For this review, take the finished solid that the model builds, in its own axes (mm). Face numbers are marked on the shaded views. Coordinates: 2 decimals unless noted, no trailing zeros. Loops run counter-clockwise (first coordinate to the right, second up) from the corner with the lowest first, then second, coordinate; pieces in that order, holes last. Notation, with made-up numbers: M 62,40 L 95,40 A33 ccw 95,75 Z; hole C 58,-25 d10. An arc over 180 degrees is marked long. Use one line per item in the form item = value.
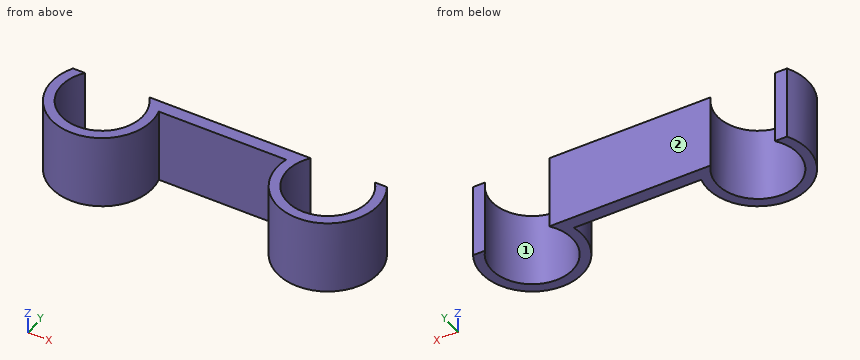
Autodesk Fusion 360 part; units mm, degrees
sketch "スケッチ1" plane through (0, 0, 0) normal (0, 0, 1) x (1, 0, 0)
  arc A0 (-11.5217, 2) -> (-4.0754, 1) centre (-8, 0) ccw
  arc A1 (-10.5617, 2) -> (-5.4383, 2) centre (-8, 0) ccw
  line L0 (-11.5217, 2) -> (-10.5617, 2)
  line L1 (-6, 1) -> (-4.9077, 1)
  line L2 (-4.0754, 1) -> (6.0754, 1)
  arc A2 (6.0754, 1) -> (13.5217, 2) centre (10, 0) ccw
  arc A3 (7.4383, 2) -> (12.5617, 2) centre (10, 0) ccw
  line L3 (-5.4383, 2) -> (7.4383, 2)
  line L4 (12.5617, 2) -> (13.5217, 2)
  dimension "d7" = 6.5
  dimension "d8" = 6.5
extrude "押し出し3" add sketch "スケッチ1" along normal blind 6
extrude "押し出し2" [suppressed]
1. Consider section D-D on x = 10. Write out the cut boundary in (y, z).
Computed values:
outline = M -4.05,0 L -3.25,0 L -3.25,6 L -4.05,6 Z
2. Draft analysis for pull direction X (two halves, no side actions). For the marked faces 1 and 2, state which applies: +X half, -X half, draft (parallel to the pull), parting line (faces both ways), or undercut.
Computed values:
face_1 = undercut
face_2 = draft
3. Consider section C-C on y = 1.5. Write out the cut boundary in (x, z), plus the area to 3 significant figures.
Computed values:
outline = M -11.76,0 L -10.88,0 L -10.88,6 L -11.76,6 Z; M -5.12,0 L 7.12,0 L 7.12,6 L -5.12,6 Z; M 12.88,0 L 13.76,0 L 13.76,6 L 12.88,6 Z
area = 83.9 mm2
4. Wall thickness on line 1 along X through (y, z) = (0, 4.8); line 2 along X through (y, z) = (-2.5, 3.25); line 3 along X through (y, z) = (1.5, 3.5): over which ranges is each line inside the solid? List them lowest first. Write a range as from..to.
Computed values:
line_1 = -12.05..-11.25, -4.75..-3.95, 5.95..6.75, 13.25..14.05
line_2 = -11.19..-10.08, -5.92..-4.81, 6.81..7.92, 12.08..13.19
line_3 = -11.76..-10.88, -5.12..7.12, 12.88..13.76
5. Consider section A-A on y = 0. Write out the cut boundary in (x, z).
Computed values:
outline = M -12.05,0 L -11.25,0 L -11.25,6 L -12.05,6 Z; M -4.75,0 L -3.95,0 L -3.95,6 L -4.75,6 Z; M 5.95,0 L 6.75,0 L 6.75,6 L 5.95,6 Z; M 13.25,0 L 14.05,0 L 14.05,6 L 13.25,6 Z
6. Consider section B-B on z = 2.5. Write out the cut boundary in (x, y).
Computed values:
outline = M -11.52,2 A4.05 ccw long -4.08,1 L 6.08,1 A4.05 ccw long 13.52,2 L 12.56,2 A3.25 cw long 7.44,2 L -5.44,2 A3.25 cw long -10.56,2 Z
7. For pin 1 Ø2 at (x, z) = (2, 4) entering from -Y; pin 2 Ø2 at (y, z) = (0.5, 4) entering from +X, all flat-tipped, find the tip position at first contact; note any pin that passes through.
Computed values:
pin_1 = 1
pin_2 = 14.05
